```python
from build123d import *

# Parameters (mm, degrees)
F1_DEPTH = 2


with BuildPart() as f1:
    # F0 (on Top) → F1 (new body)
    with BuildSketch(Plane.XY):
        with BuildLine():
            Line((5.169261, 12.4797), (0, 0))
            Line((0, 0), (-5.169261, 12.4797))
            ThreePointArc((-5.169261, 12.4797), (-6.505618, 13.372626), (-7.841976, 12.4797))
            Line((-7.841976, 12.4797), (-12.24587, 1.847759))
            ThreePointArc((-12.24587, 1.847759), (-11.704674, 0.541196), (-10.398111, 1.082392))
            Line((-10.398111, 1.082392), (-6.505618, 10.4797))
            Line((-6.505618, 10.4797), (-2.164784, 0))
            ThreePointArc((-2.164784, 0), (0, -2.164784), (2.164784, 0))
            Line((2.164784, 0), (6.505618, 10.4797))
            Line((6.505618, 10.4797), (10.398111, 1.082392))
            ThreePointArc((10.398111, 1.082392), (10.939307, 0.541196), (11.704674, 0.541196))
            ThreePointArc((11.704674, 0.541196), (12.24587, 1.082392), (12.24587, 1.847759))
            Line((12.24587, 1.847759), (7.841976, 12.4797))
            ThreePointArc((7.841976, 12.4797), (6.505618, 13.372626), (5.169261, 12.4797))
        make_face()
    extrude(amount=F1_DEPTH)


solid = f1.part
```
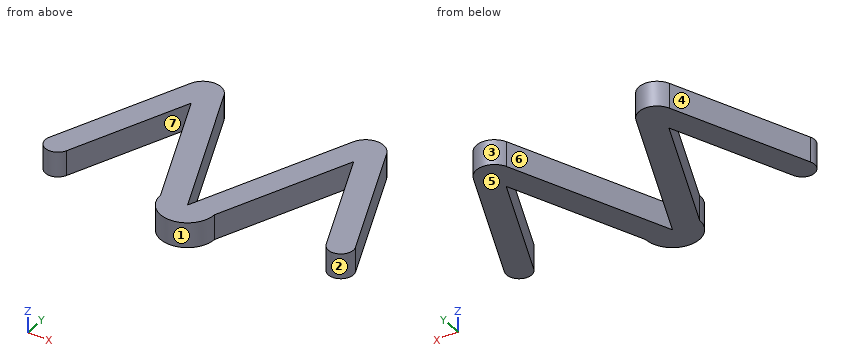
Verification items for the finished model (mm, model axes). Face numbers are marked on the shaded views. A direction names the side the tool comes from. Coordinates: 2 decimals unless noted, no trailing zeros. Loops run counter-clockwise (first coordinate to the right, second up) from the corner with the lowest first, then second, coordinate; pieces in that order, holes last. Notation, with made-up numbers: (63.25, -34.5) -> (96.25, -34.5) arc R22 cw to (96.25, -17.5) -> close; hole circle Ø11 at (-35, 66.25). An arc over 180 degrees is marked (long way). Answer in a Markdown table with one row per item.
1) Section check D-D (x = -9.75). Record the cut outline in (y, z), and give its area (3 significant figures).
The answers:
| item | result |
|---|---|
| outline | (2.65, 0) -> (7.87, 0) -> (7.87, 2) -> (2.65, 2) -> close |
| area | 10.5 mm2 |
2) Draft check along X on the marked faces 1, 2, 3 and 4. Enter one of: released by +X, released by -X, zero draft, split by the parting line, or undercut.
The answers:
| item | result |
|---|---|
| face 1 | split by the parting line |
| face 2 | undercut |
| face 3 | undercut |
| face 4 | released by -X |
3) Section check A-A (y = 4.5). Record the cut outline in (x, z), and give its area (3 significant figures).
The answers:
| item | result |
|---|---|
| outline | (-11.15, 0) -> (-8.98, 0) -> (-8.98, 2) -> (-11.15, 2) -> close; (-4.03, 0) -> (-1.86, 0) -> (-1.86, 2) -> (-4.03, 2) -> close; (1.86, 0) -> (4.03, 0) -> (4.03, 2) -> (1.86, 2) -> close; (8.98, 0) -> (11.15, 0) -> (11.15, 2) -> (8.98, 2) -> close |
| area | 17.3 mm2 |
4) Section check B-B (z = 1.1). Record the cut outline in (x, y), and give its area (3 significant figures).
The answers:
| item | result |
|---|---|
| outline | (-12.25, 1.85) arc R1 ccw to (-10.4, 1.08) -> (-6.51, 10.48) -> (-2.16, 0) arc R2.16 ccw to (2.16, 0) -> (6.51, 10.48) -> (10.4, 1.08) arc R1 ccw to (12.25, 1.85) -> (7.84, 12.48) arc R1.45 ccw to (5.17, 12.48) -> (0, 0) -> (-5.17, 12.48) arc R1.45 ccw to (-7.84, 12.48) -> close |
| area | 112 mm2 |
5) Access from +Z, -Z, +X, -X, +Y, -Y to the whole of each face (thin tool, end or side, straight path). Record for the marked faces 5, 6 and 7.
The answers:
| item | result |
|---|---|
| face 5 | -Z, +X, -X, +Y, -Y |
| face 6 | +Z, -Z, +Y |
| face 7 | +Z, -Z, -Y |
6) Section check C-C (y = 11.25). Record the cut outline in (x, z).
The answers:
| item | result |
|---|---|
| outline | (-8.35, 0) -> (-4.66, 0) -> (-4.66, 2) -> (-8.35, 2) -> close; (4.66, 0) -> (8.35, 0) -> (8.35, 2) -> (4.66, 2) -> close |
7) Scan lines: line 1 along X through (y, z) = (4, 1.75); line 2 along X through (y, z) = (6, 1.2); line 3 along X through (y, z) = (12.25, 1.65). Record each from-to range of solid material in increasing order. Write a range as from..to.
The answers:
| item | result |
|---|---|
| line 1 | x = -11.35..-9.19, -3.82..-1.66, 1.66..3.82, 9.19..11.35 |
| line 2 | x = -10.53..-8.36, -4.65..-2.49, 2.49..4.65, 8.36..10.53 |
| line 3 | x = -7.94..-5.07, 5.07..7.94 |
